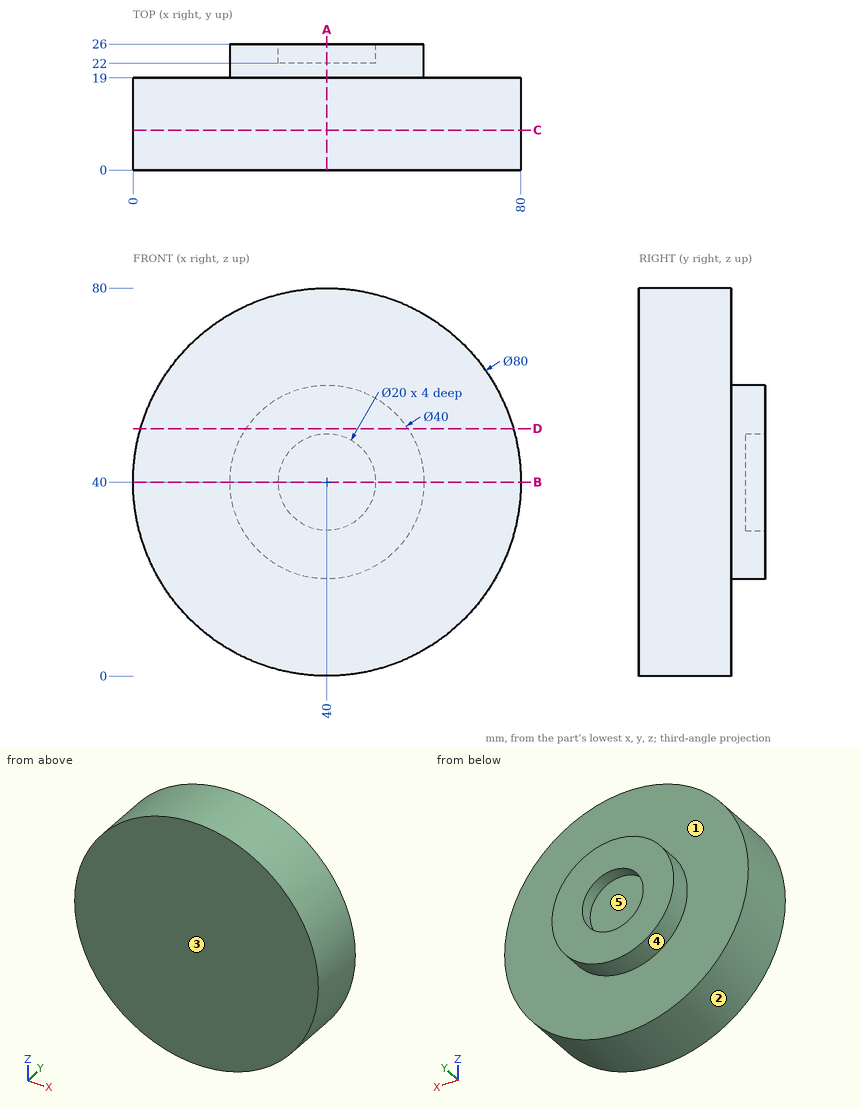
Geometry: see drawing. Coordinates: mm, zero at the bounding-box minimum. A direction names the side the tool comes from. Coordinates: 2 decimals unless noted, no trailing zeros. Loops run counter-clockwise (first coordinate to the right, second up) from the corner with the lowest first, then second, coordinate; pieces in that order, holes last. Notation, with made-up numbers: (-16, -28) - (-8, -28) arc R20 cw to (-8, -3) - close; hole circle Ø2 at (-34.5, 69). An arc over 180 degrees is marked (long way). Answer as CSV lines item,"result".
1. Ray query, line 1 (Z direction, x = 40, y = 24.8); line 2 (Y direction, x = 38, z = 65). Return the intervals inside material, ascending.
Established:
line 1,"z = 20 to 30, 50 to 60"
line 2,"y = 0 to 19"
2. Section C-C (y = 8.25). Return loops of the section in (x, z), then the cut area to 3 significant figures.
Established:
outline,"circle Ø80 at (40, 40)"
area,"5,030 mm2"
3. Reachability of the marked faces 1 and 2 from +Z, -Z, +X, -X, +Y, -Y: full face, straight path, thin tool, end or side. Return the list, or none.
Established:
face 1,"+Y"
face 2,"+Y, -Y"
4. Mould query, pull axis Z, two halves, no side actions, for the marked faces 3, 4 and 5. Classes: released by +Z, released by -Z, zero draft, split by the parting line, or undercut.
Established:
face 3,"zero draft"
face 4,"split by the parting line"
face 5,"undercut"
5. Section A-A (x = 40). Return loops of the section in (y, z).
Established:
outline,"(0, 0) - (19, 0) - (19, 20) - (26, 20) - (26, 30) - (22, 30) - (22, 50) - (26, 50) - (26, 60) - (19, 60) - (19, 80) - (0, 80) - close"
6. Section B-B (z = 40). Return loops of the section in (x, y), then the cut area to 3 significant figures.
Established:
outline,"(0, 0) - (80, 0) - (80, 19) - (60, 19) - (60, 26) - (50, 26) - (50, 22) - (30, 22) - (30, 26) - (20, 26) - (20, 19) - (0, 19) - close"
area,"1,720 mm2"
7. Contact query for flat-ended pins moving along their axis: pin 1 (12 mm diameter, centred on y = 3.5, z = 25.5, fed in from +X); pin 2 (12 mm diameter, centred on x = 42, z = 8.5, fed in from +Y); pin 3 (5 mm diameter, centred on x = 51, y = 8.5, fed in from +Z). Output: stop coordinate, or through.
Established:
pin 1,"stops at x = 79.09"
pin 2,"stops at y = 19"
pin 3,"stops at z = 79.09"
8. Section D-D (z = 51). Return loops of the section in (x, y).
Established:
outline,"(1.54, 0) - (78.46, 0) - (78.46, 19) - (56.7, 19) - (56.7, 26) - (23.3, 26) - (23.3, 19) - (1.54, 19) - close"
